Can you work these out from the model? Positions are in its coordinate system, mm. Give positions to 0.01 mm unless a question says otherwise; leave off trailing zeros. Write each loop counter-clockwise with the first axis right and the second up, starting at its lowest first coordinate (ties: lowest second). Pieces come first, ordered by that corner, then holes.
```python
from build123d import *

# Parameters (mm, degrees)
SKETCH1_R        = 5
BASEHEAD_DEPTH   = 3.9
BASEHEAD_DRAFT   = -5
SKETCH8_W        = 20
SKETCH8_H        = 3
SOCKET_DEPTH     = 2
HEADFILLET2_R    = 1
LPATTERN10_COUNT = 31
LPATTERN10_PITCH = 0.6498


with BuildPart() as part:
    # Sketch1 → BaseHead (with draft: the straight prism first)
    with BuildSketch(Plane(origin=(3.9, 0, 0), x_dir=(0, 0, -1), z_dir=(1, 0, 0))):
        Circle(SKETCH1_R)
    extrude(amount=-BASEHEAD_DEPTH)
    # BaseHead: the draft: its side faces are tilted about the plane it starts from
    basehead_sides = [part.faces().sort_by_distance(p)[0] for p in [
        (1.95, 0, 5),
    ]]
    draft(basehead_sides, Plane(origin=(3.9, 0, 0), x_dir=(0, 0, -1), z_dir=(1, 0, 0)), BASEHEAD_DRAFT)

    # Sketch8 → Revolve1 (revolve)
    with BuildSketch(Plane.XY, mode=Mode.PRIVATE) as revolve1_sk:
        with Locations((13.9, 1.5)):
            Rectangle(SKETCH8_W, SKETCH8_H)
    revolve(revolve1_sk.sketch.rotate(Axis((0, 0, 0), (1, 0, 0)), 90), axis=Axis((0, 0, 0), (1, 0, 0)))

    # Sketch4 → Socket (cut)
    with BuildSketch(Plane(origin=(0, 0, 0), x_dir=(0, 0, -1), z_dir=(1, 0, 0))):
        with BuildLine():
            add(Edge.make_bspline(
                [(1.0375, 1.797002713), (1.436538462, 1.56661775), (2.394230769, 1.382309779), (1.915384615, 0), (2.394230769, -1.382309779), (0.957692308, -1.658771735), (0, -2.764619558), (-0.957692308, -1.658771735), (-2.394230769, -1.382309779), (-1.915384615, 0), (-2.394230769, 1.382309779), (-0.957692308, 1.658771735), (0, 2.764619558), (0.638461538, 2.027387676), (1.0375, 1.797002713)],
                knots=[0, 0, 0, 0, 0.083333333, 0.166666667, 0.25, 0.333333333, 0.416666667, 0.5, 0.583333333, 0.666666667, 0.75, 0.833333333, 0.916666667, 1, 1, 1, 1], degree=3))
        make_face()
    extrude(amount=SOCKET_DEPTH, mode=Mode.SUBTRACT)

    # Sketch5 → Cut-Loft1 section 0
    with BuildSketch(Plane.ZY.offset(-2), mode=Mode.PRIVATE) as cut_loft1_s0:
        with BuildLine():
            add(Edge.make_bspline(
                [(-1.0375, 1.797002713), (-1.436538462, 1.56661775), (-2.394230769, 1.382309779), (-1.915384615, 0), (-2.394230769, -1.382309779), (-0.957692308, -1.658771735), (0, -2.764619558), (0.957692308, -1.658771735), (2.394230769, -1.382309779), (1.915384615, 0), (2.394230769, 1.382309779), (0.957692308, 1.658771735), (0, 2.764619558), (-0.638461538, 2.027387676), (-1.0375, 1.797002713)],
                knots=[0, 0, 0, 0, 0.083333333, 0.166666667, 0.25, 0.333333333, 0.416666667, 0.5, 0.583333333, 0.666666667, 0.75, 0.833333333, 0.916666667, 1, 1, 1, 1], degree=3))
        make_face()
    loft([Vertex(2.666666667, 0, 0), cut_loft1_s0.sketch], mode=Mode.SUBTRACT)

    # HeadFillet2
    headfillet2_edges = [part.edges().sort_by_distance(p)[0] for p in [
        (0, 0, 4.658794212),
    ]]
    fillet(headfillet2_edges, radius=HEADFILLET2_R)

    # Sketch9 → Cut-Revolve10 (revolve, cut)
    with BuildSketch(Plane.XY, mode=Mode.PRIVATE) as cut_revolve10_sk:
        Polygon((23.9, 2.531047244), (24.17075, 3), (24.17075, 3.5415), (23.62925, 3.5415), (23.62925, 3), align=None)
    cut_revolve10 = revolve(cut_revolve10_sk.sketch.rotate(Axis((0, 0, 0), (1, 0, 0)), 90), axis=Axis((0, 0, 0), (1, 0, 0)), mode=Mode.SUBTRACT)

    # LPattern10: Cut-Revolve10 ×31
    with Locations(*[(-i * LPATTERN10_PITCH, 0, 0) for i in range(1, LPATTERN10_COUNT)]):
        add(cut_revolve10, mode=Mode.SUBTRACT)


solid = part.part
```
1) For pin 1 Ø1.5 at (x, y) = (18.5, -0.5) entering from -Z; pin 2 Ø1.5 at (x, z) = (11, -3) entering from -Y; pin 3 Ø4 at (x, y) = (16, 2.5) entering from +Z, each with a flat end and sliding along its axis, tell me the tip position at first contact or that it passes through.
Values follow:
pin 1: stops at z = -3
pin 2: stops at y = -1.96
pin 3: stops at z = 2.96
2) Please list where these lines run through material, in increasing order: L1, parallel to X at y = 3.25, z = 1.75; L2, parallel to Z at x = 12.25, y = -1.25; L3, parallel to Y at x = 7.5, z = -0.5.
Values follow:
L1: x = 0 to 3.9
L2: z = -2.29 to 2.29
L3: y = -2.75 to 2.75
3) Suppose I cut it at A-A on x = 3. Write out the boundary of the cut face in (y, z).
Values follow:
outline: circle Ø9.84 at (0, 0)
